Input: part model. Units: mm. Frame: model coordinates. A direction names the side the tool comes from. Round coordinates to 2 decimals unless told otherwise and drop trailing zeros. Loops run counter-clockwise (first coordinate to the right, second up) from the corner with the lowest first, then second, coordinate; pieces in that order, holes last. Notation, with made-up numbers: (54.25, 80.25) - (95.25, 80.25) arc R11 cw to (95.25, 84.25) - close; hole circle Ø11 at (-40, 84.25). An arc over 180 degrees is marked (long way). Write each question's results on one line, items separated by ' | '.
from build123d import *

# Parameters (mm, degrees)
BOSS_EXTRUDE1_DEPTH = 6
SKETCH2_W           = 10
SKETCH2_H           = 10
BOSS_EXTRUDE2_DEPTH = 12
SKETCH3_R           = 1.75
CUT_EXTRUDE1_DEPTH  = 36.944401511
CUT_EXTRUDE2_DEPTH  = 3


with BuildPart() as part:
    # Sketch1 → Boss-Extrude1 (new body)
    with BuildSketch(Plane(origin=(0, 0, 0), x_dir=(1, 0, 0), z_dir=(0, 1, 0))):
        Polygon((0, 0), (0, 22), (10, 22), (10, 10), (22, 10), (22, 0), align=None)
    extrude(amount=BOSS_EXTRUDE1_DEPTH)

    # Sketch2 → Boss-Extrude2 (add)
    with BuildSketch(Plane(origin=(0, 6, 0), x_dir=(1, 0, 0), z_dir=(0, 1, 0))):
        with Locations((5, 5)):
            Rectangle(SKETCH2_W, SKETCH2_H)
    extrude(amount=BOSS_EXTRUDE2_DEPTH)

    # Sketch3 → Cut-Extrude1 (cut, through all)
    with BuildSketch(Plane(origin=(0, 18, 0), x_dir=(1, 0, 0), z_dir=(0, 1, 0))):
        with Locations(Location((5, 5, 0), (0, 0, 270))):
            Circle(SKETCH3_R)
    extrude(amount=-CUT_EXTRUDE1_DEPTH, mode=Mode.SUBTRACT)

    # Sketch4 → Cut-Extrude2 (cut)
    with BuildSketch(Plane.XZ):
        Polygon((1.824573519, -5), (3.41228676, -7.75), (6.58771324, -7.75), (8.175426481, -5), (6.58771324, -2.25), (3.41228676, -2.25), align=None)
    extrude(amount=-CUT_EXTRUDE2_DEPTH, mode=Mode.SUBTRACT)


solid = part.part
1. Line query: line 1 (X direction, y = 15.25, z = -5); line 2 (Z direction, x = 1.5, y = 9.5); line 3 (Y direction, x = 5.5, z = -18.25). Output: solid intervals per line, ascending. Write a range as [from, to].
Answer:
line 1: [0, 3.25], [6.75, 10] | line 2: [-10, 0] | line 3: [0, 6]
2. Section query D-D, the plane x = 11.75. Output: boundary loops of the cut face in (y, z).
Answer:
outline: (0, -10) - (6, -10) - (6, 0) - (0, 0) - close
3. Mould query, pull axis Z, two halves, no side actions, for faces 1 (the flat face through (5, 3, -22)), 2 (the flat face through (10, 3, -16)), 3 (the flat face through (5, 1, -7.75)). Classes: pulls with the +Z half, pulls with the -Z half, needs draft (parallel to the pull), parting line crosses it, or undercut.
Answer:
face 1: pulls with the -Z half | face 2: needs draft | face 3: undercut
4. Section query B-B, the plane x = 5. Output: boundary loops of the cut face in (y, z).
Answer:
outline: (0, -22) - (6, -22) - (6, -10) - (18, -10) - (18, -6.75) - (3, -6.75) - (3, -7.75) - (0, -7.75) - close; (0, -2.25) - (3, -2.25) - (3, -3.25) - (18, -3.25) - (18, 0) - (0, 0) - close
5. Contact query for flat-ended pins moving along their axis: pin 1 (6 mm diameter, centred on x = 5.5, z = -4.5, fed in from -Y); pin 2 (6.5 mm diameter, centred on x = 15.5, y = 2.5, fed in from -Z); pin 3 (11 mm diameter, centred on x = 18.5, z = -7.5, fed in from +Y); pin 4 (4 mm diameter, centred on y = 2.5, z = -16, fed in from +X). Output: stop coordinate, or through.
Answer:
pin 1: y = 0 | pin 2: z = -10 | pin 3: y = 6 | pin 4: x = 10
6. Set-up query: faces 4 (the flat face through (10, 12, -5)), 5 (the flat face through (5, 12, -10)), 6 (the flat face through (5, 1, -2.25)). Return all of +Z, -Z, +X, -X, +Y, -Y with unobstructed straight access to the full face (end or side cutting, diameter ignored); none if empty.
Answer:
face 4: +Z, -Z, +X, +Y | face 5: -Z, +X, -X, +Y | face 6: -Y
7. Section query C-C, the plane z = -8.75. Output: boundary loops of the cut face in (x, y), plus the area to 3 significant figures.
Answer:
outline: (0, 0) - (22, 0) - (22, 6) - (10, 6) - (10, 18) - (0, 18) - close | area: 252 mm^2
8. Section query A-A, the plane y = 4.75. Output: boundary loops of the cut face in (x, z).
Answer:
outline: (0, -22) - (10, -22) - (10, -10) - (22, -10) - (22, 0) - (0, 0) - close; hole circle Ø3.5 at (5, -5)
